```python
from build123d import *

# Parameters (mm, degrees)
CROQUIS1_R              = 1.743
CROQUIS1_R_2            = 1.745
SALIENTE_EXTRUIR1_DEPTH = 8.5


with BuildPart() as part:
    # Croquis1 → Saliente-Extruir1 (new body)
    with BuildSketch(Plane.XY):
        with BuildLine():
            Line((-8.694, 5), (0, 5))
            ThreePointArc((0, 5), (5, 0), (0, -5))
            Line((0, -5), (-22, -5))
            add(Edge.make_bspline(
                [(-22, -5), (-22.376114087, -5.000730995), (-23.127936381, -4.912027071), (-23.842743751, -4.662668406), (-24.18108985, -4.497)],
                knots=[0, 0, 0, 0, 0.499595813, 1, 1, 1, 1], degree=3))
            Line((-24.18108985, -4.497), (-33.082774185, -0.176))
            Line((-33.082774185, -0.176), (-34.150774185, 0.655))
            Line((-34.150774185, 0.655), (-35.235774185, 1.426))
            Line((-35.235774185, 1.426), (-36.329774185, 2.134))
            Line((-36.329774185, 2.134), (-37.433774185, 2.78))
            Line((-37.433774185, 2.78), (-38.592774185, 3.367))
            add(Edge.make_bspline(
                [(-38.592774185, 3.367), (-39.332541124, 3.73458873), (-40.463584029, 4.233674803), (-42.009779682, 4.789621338), (-43.18029785, 5.1503195), (-44.367367964, 5.455509833), (-45.571550782, 5.707001476), (-46.794958977, 5.902822636), (-48.465017773, 6.09379478), (-49.733307298, 6.151003132), (-50.584774185, 6.154)],
                knots=[0, 0, 0, 0, 0.199499465, 0.298230174, 0.396705181, 0.49521602, 0.594152289, 0.693710503, 0.79435234, 1, 1, 1, 1], degree=3))
            add(Edge.make_bspline(
                [(-50.584774185, 6.154), (-51.784512946, 6.156123129), (-52.980774185, 6.067)],
                knots=[0, 0, 0, 1, 1, 1], degree=2))
            Line((-52.980774185, 6.067), (-60.345774185, 9.189))
            Line((-60.345774185, 9.189), (-58.785774185, 12.872))
            add(Edge.make_bspline(
                [(-47.376936723, 15.389), (-48.196892042, 15.403291142), (-49.398277121, 15.379717661), (-50.970775635, 15.224558885), (-52.098811061, 15.061295448), (-53.219989961, 14.84128524), (-54.336112455, 14.567008142), (-55.4494326, 14.235014339), (-56.95056509, 13.707761437), (-58.056017514, 13.22696924), (-58.785774185, 12.872)],
                knots=[0, 0, 0, 0, 0.208580678, 0.30512865, 0.401665607, 0.498317749, 0.595560953, 0.693826211, 0.793634588, 1, 1, 1, 1], degree=3))
            add(Edge.make_bspline(
                [(-14.621, 5.599), (-15.563222131, 5.781119084), (-17.011007703, 6.120848832), (-18.989445264, 6.684731463), (-20.635507849, 7.208092626), (-22.439927245, 7.83467175), (-24.540120329, 8.619913648), (-27.091397312, 9.631396334), (-29.90077475, 10.772491334), (-32.584990491, 11.839895748), (-34.794603661, 12.665403671), (-36.602182307, 13.292835375), (-38.193000796, 13.796531357), (-39.671884667, 14.211722291), (-41.068328907, 14.576337495), (-42.402463198, 14.85165039), (-43.69443221, 15.078308418), (-45.342048595, 15.292337563), (-46.568508645, 15.371828774), (-47.376936723, 15.389)],
                knots=[0, 0, 0, 0, 0.083834458, 0.129855591, 0.179713331, 0.234726598, 0.296726991, 0.375600314, 0.474504455, 0.561662864, 0.627975282, 0.680575135, 0.728822097, 0.773739203, 0.814774439, 0.854888969, 0.892720603, 0.929358167, 1, 1, 1, 1], degree=3))
            Line((-14.621, 5.599), (-13.161, 5.346))
            Line((-13.161, 5.346), (-11.763, 5.166))
            Line((-11.763, 5.166), (-10.416, 5.05))
            Line((-10.416, 5.05), (-9.11, 5))
            Line((-9.11, 5), (-8.694, 5))
        make_face()
        Circle(CROQUIS1_R, mode=Mode.SUBTRACT)
        with Locations((-22, 0)):
            Circle(CROQUIS1_R_2, mode=Mode.SUBTRACT)
    extrude(amount=SALIENTE_EXTRUIR1_DEPTH)


solid = part.part
```
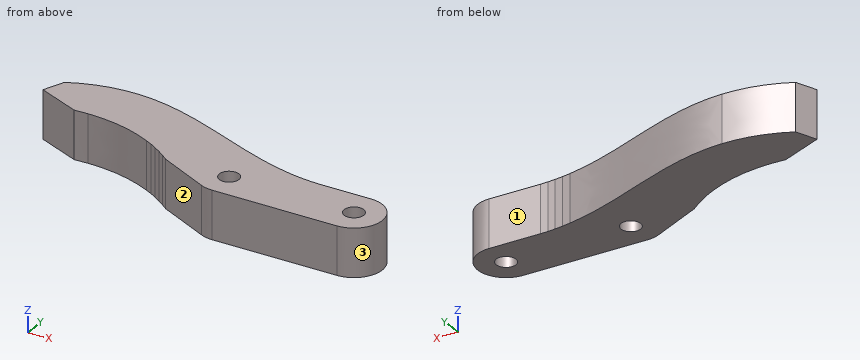
Input: part model. Units: mm. Frame: model coordinates. Face numbers are marked on the shaded views. Give positions to 0.01 mm unless a question says otherwise; leave off trailing zeros. Order: outer loops, then holes, each group sorted by start corner. A loop starts at its lowest first (then second) coordinate and runs counter-clockwise, first axis right, second up. Notation, with made-up numbers: (-2.75, 22) - (12.25, 22) arc R12 ccw to (12.25, 40) - close; hole circle Ø5 at (-27.5, 56). An arc over 180 degrees is marked (long way). Put each result on its own line as item: value.
Item 1: Section query A-A, the plane z = 7. Count the separate pieces of the cut face and the enclosed holes in it, then the cut area to 3 significant figures.
Found:
separate pieces: 1
enclosed holes: 2
area: 636 mm^2
Item 2: Contact query for flat-ended pins moving along their axis: pin 1 (3 mm diameter, centred on x = -22, y = 0, fed in from +Z); pin 2 (5 mm diameter, centred on x = -28, z = 1.5, fed in from +Y); pin 3 (4 mm diameter, centred on x = -6, z = 5, fed in from +Y). Output: stop coordinate, or through.
Found:
pin 1: passes through
pin 2: stops at y = 11.01
pin 3: stops at y = 5
Item 3: Draft query along X for the marked faces 1, 2 and 3. Return one class per face: +X half, -X half, draft (parallel to the pull), parting line (faces both ways), or undercut.
Found:
face 1: draft
face 2: -X half
face 3: +X half
Item 4: Section query B-B, the plane x = -14. Return loops of the section in (y, z), then the cut area to 3 significant figures.
Found:
outline: (-5, 0) - (5.49, 0) - (5.49, 8.5) - (-5, 8.5) - close
area: 89.2 mm^2
Item 5: Ray query, L1, parallel to X at y = -1.25, z = 1.75; L2, parallel to X at y = -3.25, z = 1.25; L3, parallel to Y at x = -41.5, z = 6. Return the intervals inside material, ascending. Write a range as from..to.
Found:
L1: x = -30.87..-23.22, -20.78..-1.21, 1.21..4.84
L2: x = -26.75..3.8
L3: y = 4.6..14.66
